from build123d import *

# Parameters (mm, degrees)
BOSS_EXTRUDE1_DEPTH = 10


with BuildPart() as part:
    # Sketch1 → Boss-Extrude1 (new body)
    with BuildSketch(Plane.XY):
        with BuildLine():
            ThreePointArc((2.47842575, -12.251832753), (-1.137379909, 12.448147129), (-0.217037467, -12.498115647))
            add(Edge.make_bspline(
                [(-0.217037467, -12.498115647), (0.103518304, -14.995056083), (1.115421548, -17.260389343)],
                knots=[0, 0, 0, 1, 1, 1], degree=2))
            add(Edge.make_bspline(
                [(1.115421548, -17.260389343), (0.434564651, -18.108574327), (0, -17.447731212)],
                knots=[0, 0, 0, 1, 1, 1], degree=2))
            add(Edge.make_bspline(
                [(0, -17.447731212), (-1.091166652, -16.283532634), (-1.609840573, -14.937630884), (-1.556021763, -13.410025961)],
                knots=[0, 0, 0, 0, 0.825397526, 0.825397526, 0.825397526, 0.825397526], degree=3))
            ThreePointArc((-1.556021763, -13.410025961), (-1.523641622, 13.413743557), (4.524014275, -12.71940623))
            add(Edge.make_bspline(
                [(4.524014275, -12.71940623), (3.253229228, -14.746642768), (8.549206323, -14.842102086), (5.577194292, -16.538556843)],
                knots=[0, 0, 0, 0, 1, 1, 1, 1], degree=3))
            add(Edge.make_bspline(
                [(2.47842575, -12.251832753), (1.654957901, -15.727340902), (5.577194292, -16.538556843)],
                knots=[0, 0, 0, 1, 1, 1], degree=2))
        make_face()
    extrude(amount=BOSS_EXTRUDE1_DEPTH)


solid = part.part
For this review, take the finished solid that the model builds, in its own axes (mm). Give positions to 0.01 mm unless a question says otherwise; leave off trailing zeros. Order: outer loops, then holes, each group sorted by start corner. A loop starts at its lowest first (then second) coordinate and runs counter-clockwise, first axis right, second up. Notation, with made-up numbers: M 0.5,-19 L 36.5,-19 A36 cw 36.5,20 Z; hole C 27,20.25 d2. An arc over 180 degrees is marked long. Answer in a Markdown table with one row per item. Add a question column.
(1) Consider section A-A on y = 0. State the section outline as (x, z) points.
(2) Consider section B-B on x = 7.5. State the section outline as (y, z) points.
(3) Mouldability with a two-part tool opening along X and no side actions: class faces 1 (the face through (-0.608, 12.485, 4.93)), 2 (the face through (5, -12, 0)), 3 (the face through (-2.07, 13.34, 4.93)) as +X half, -X half, draft (parallel to the pull), parting line (faces both ways), or undercut.
(4) Wall thickness on probe 1 along Y at (x, z) = (5, 2.25); probe 2 along X at (y, z) = (0, 5.5); probe 3 along X at (y, z) = (9, 2.25): over which ranges is each line inside the solid? List them lowest first. Write a range as [from, to].
(5) For pin 1 (4 mm diameter, centred on x = -4.5, z = 8.5, fed in from +Y); pin 2 (3 mm diameter, centred on x = 7, z = 7.5, fed in from -Y); pin 3 (6 mm diameter, centred on x = -10, y = -10.5, fed in from +Z); pin 4 (10 mm diameter, centred on x = -7, y = 0, fed in from +Z), all flat-tipped, find the tip position at first contact; note any pin that passes through.
Evaluation:
| question | item | result |
|---|---|---|
| 1 | outline | M -13.5,0 L -12.5,0 L -12.5,10 L -13.5,10 Z; M 12.5,0 L 13.5,0 L 13.5,10 L 12.5,10 Z |
| 2 | outline | M -11.22,0 L -10,0 L -10,10 L -11.22,10 Z; M 10,0 L 11.22,0 L 11.22,10 L 10,10 Z |
| 3 | face 1 | undercut |
| 3 | face 2 | draft |
| 3 | face 3 | parting line |
| 4 | probe 1 | y = [-16.4, -14.31], [-12.54, -11.46], [11.46, 12.54] |
| 4 | probe 2 | x = [-13.5, -12.5], [12.5, 13.5] |
| 4 | probe 3 | x = [-10.06, -8.67], [8.67, 10.06] |
| 5 | pin 1 | stops at y = 13.27 |
| 5 | pin 2 | stops at y = -16.54 |
| 5 | pin 3 | stops at z = 10 |
| 5 | pin 4 | passes through |
